Can you work these out from the model? Positions are in its coordinate system, mm. A direction names the side the tool comes from. Round coordinates to 2 decimals unless told otherwise and drop trailing zeros. Order: outer loops, then holes, each group sorted by start corner. A loop starts at its lowest first (then second) coordinate and runs counter-clockwise, first axis right, second up. Notation, with made-up numbers: M 29.25,24.25 L 33.25,24.25 A17 ccw 33.25,32.25 Z; hole C 76,-28 d4. An arc over 180 degrees is marked long. Answer as a JSON object with one key per item and string values. Group by question number.
Autodesk Inventor part; units mm, degrees
ref_plane "YZ Plane" through (0, 0, 0) normal (1, 0, 0) x (0, 1, 0)
ref_plane "XZ Plane" through (0, 0, 0) normal (0, 1, 0) x (-1, 0, 0)
ref_plane "XY Plane" through (0, 0, 0) normal (0, 0, 1) x (1, 0, 0)
sketch "Sketch1" plane through (0, 0, 0) normal (0, 0, 1) x (1, 0, 0)
  line L0 (0, 0) -> (0, 52.9336)
  line L1 (0, 52.9336) -> (193.1614, 63.023)
  line L2 (193.1614, 63.023) -> (0, 0)
  dimension "d0" = 52.9336
  dimension "d34" = 15.08
  dimension "d48" = 92.99
extrude "Extrusion1" add sketch "Sketch1" along normal blind 3.175
sketch "Sketch5" plane through (0, 0, 3.175) normal (0, 0, 1) x (1, 0, 0)
  line L0 (0, 52.9336) -> (0, 0)
  line L1 (193.1614, 63.023) -> (0, 52.9336)
  line L2 (0, 30.2768) -> (-3.175, 30.2768)
  line L3 (-3.175, 30.2768) -> (-3.175, 22.6568)
  line L4 (-3.175, 22.6568) -> (0, 22.6568)
  line L5 (0, 22.6568) -> (0, 30.2768)
  line L6 (100.3855, 58.177) -> (100.2199, 61.3477)
  line L7 (100.2199, 61.3477) -> (92.6103, 60.9502)
  line L8 (92.6103, 60.9502) -> (92.7759, 57.7795)
  line L9 (92.7759, 57.7795) -> (100.3855, 58.177)
  line L10 (0, 0) -> (193.1614, 63.023)
  line L11 (100.2028, 32.6933) -> (101.1876, 29.6749)
  line L12 (101.1876, 29.6749) -> (93.9434, 27.3113)
  line L13 (93.9434, 27.3113) -> (92.9586, 30.3297)
  line L14 (92.9586, 30.3297) -> (100.2028, 32.6933)
  point P0 (0, 26.4668)
  point P1 (96.5807, 57.9783)
  point P2 (96.5807, 31.5115)
  dimension "d36" = 7.62
  dimension "d37" = 3.81
  dimension "d38" = 3.175
  dimension "d39" = 3.81
  dimension "d40" = 7.62
  dimension "d41" = 3.175
  dimension "d42" = 3.81
  dimension "d44" = 7.62
  dimension "d45" = 3.175
extrude "Extrusion5" add sketch "Sketch5" against normal blind 3.175 contours L0 L4 L3 L2 | L8 L7 L6 L1 | L10 L11 L12 L13
sketch "Sketch6" plane through (0, 0, 3.175) normal (0, 0, 1) x (1, 0, 0)
  line L0 (0, 0) -> (0, 22.6568)
  line L1 (0, 22.6568) -> (-3.175, 22.6568)
  line L2 (-3.175, 22.6568) -> (-3.175, 30.2768)
  line L3 (-3.175, 22.6568) -> (-3.175, 30.2768)
  line L4 (-3.175, 30.2768) -> (0, 30.2768)
  line L5 (0, 30.2768) -> (0, 52.9336)
  line L6 (0, 30.2768) -> (0, 52.9336)
  line L7 (0, 52.9336) -> (92.7759, 57.7795)
  line L8 (92.7759, 57.7795) -> (0, 52.9336)
  line L9 (92.7759, 57.7795) -> (92.6103, 60.9502)
  line L10 (92.6103, 60.9502) -> (100.2199, 61.3477)
  line L11 (92.6103, 60.9502) -> (100.2199, 61.3477)
  line L12 (100.2199, 61.3477) -> (100.3855, 58.177)
  line L13 (100.3855, 58.177) -> (193.1614, 63.023)
  line L14 (100.3855, 58.177) -> (193.1614, 63.023)
  line L15 (193.1614, 63.023) -> (100.2028, 32.6933)
  line L16 (101.1876, 29.6749) -> (93.9434, 27.3113)
  line L17 (100.2028, 32.6933) -> (101.1876, 29.6749)
  line L18 (101.1876, 29.6749) -> (93.9434, 27.3113)
  line L19 (93.9434, 27.3113) -> (92.9586, 30.3297)
  line L20 (92.9586, 30.3297) -> (0, 0)
  line L21 (92.9586, 30.3297) -> (0, 0)
properties part number "Star Side Out" material "Wood (Birch)"
Item 1: On a 3-axis mill with a long thin cutter (end or side, diameter ignored), from which of +Z, -Z, +X, -X, +Y, -Y can I reach the whole of each face in a straight line? I mean faces 4 (the face through (100.304, 59.74, 1.61)), 5 (the face through (92.69, 59.39, 1.61)), 6 (the face through (-2, 30.277, 2)), 7 (the face through (0, 11, 2)). Say none if no direction works.
Item 2: Suppose I cut it at B-B, the plane y = 55.5. Write out the boundary of the cut face in (x, z) (3 decimals).
Item 3: I'm going to push flat-ended pins straight in: pin 1 Ø1 at (x, z) = (-2.5, 2.5) entering from +Y; pin 2 Ø1 at (y, z) = (14, 1) entering from -X. Where does each tip first touch, or does it pass through?
Item 4: If we mould it in two halves opening along X, with no side actions, what happens to faces 1 (the face through (97.62, 28.51, 1.61)), 2 (the face through (146.124, 60.566, 1.565)), 3 (the face through (96.47, 61.15, 1.61))? For each: +X half, -X half, draft (parallel to the pull), parting line (faces both ways), or undercut.
Item 5: Suppose I cut it at A-A, the plane z = 0.5. Write out the boundary of the cut face in (x, y) (1 decimal).
Item 6: I need wall thicknesses on line 1 (Y direction, x = 80, z = 2.5); line 2 (Y direction, x = 70.5, z = 2.8); line 3 (X direction, y = 31, z = 1.7). Which ranges of each line are inside material? Lowest first, please.
Item 7: Suppose I cut it at C-C, the plane x = 9. Write out the boundary of the cut face in (y, z) (3 decimals), and give its area (3 significant figures).
Computed:
{
 "1": {"face 4": "+Z, -Z, +Y", "face 5": "+Z, -Z, -X", "face 6": "+Z, -Z, -X, +Y", "face 7": "+Z, -Z, -X, -Y"},
 "2": {"outline": "M 49.134,0 L 170.104,0 L 170.104,3.175 L 49.134,3.175 Z"},
 "3": {"pin 1": "stops at y = 30.28", "pin 2": "stops at x = 0"},
 "4": {"face 1": "+X half", "face 2": "undercut", "face 3": "-X half"},
 "5": {"outline": "M -3.2,22.7 L 0,22.7 L 0,0 L 93,30.3 L 93.9,27.3 L 101.2,29.7 L 100.2,32.7 L 193.2,63 L 100.4,58.2 L 100.2,61.3 L 92.6,61 L 92.8,57.8 L 0,52.9 L 0,30.3 L -3.2,30.3 Z"},
 "6": {"line 1": "y = 26.1 to 57.11", "line 2": "y = 23 to 56.62", "line 3": "x = 0 to 100.76"},
 "7": {"outline": "M 2.936,0 L 53.404,0 L 53.404,3.175 L 2.936,3.175 Z", "area": "160 mm^2"}
}
